```python
from build123d import *

# Parameters (mm, degrees)
BOSS_EXTRUDE1_DEPTH = 609.6
SKETCH3_W           = 635.2
SKETCH3_H           = 38.1
CUT_EXTRUDE1_DEPTH  = 60


with BuildPart() as part:
    # Sketch2 → Boss-Extrude1 (new, symmetric)
    with BuildSketch(Plane.XY):
        with BuildLine():
            Line((-19.05, -19.05), (19.05, -19.05))
            Line((19.05, -19.05), (19.05, 19.05))
            Line((19.05, 19.05), (17.4625, 19.05))
            ThreePointArc((17.4625, 19.05), (16.339967985, 18.585032015), (15.875, 17.4625))
            Line((15.875, 17.4625), (15.875, -11.0998))
            ThreePointArc((15.875, -11.0998), (14.476376302, -14.476376302), (11.0998, -15.875))
            Line((11.0998, -15.875), (-17.4625, -15.875))
            ThreePointArc((-17.4625, -15.875), (-18.585032015, -16.339967985), (-19.05, -17.4625))
            Line((-19.05, -17.4625), (-19.05, -19.05))
        make_face()
    extrude(amount=BOSS_EXTRUDE1_DEPTH, both=True)

    # Sketch3 → Cut-Extrude1 (cut)
    with BuildSketch(Plane(origin=(19.05, 0, 0), x_dir=(0, 0, -1), z_dir=(1, 0, 0))):
        with Locations((292, 0)):
            Rectangle(SKETCH3_W, SKETCH3_H)
    extrude(amount=-CUT_EXTRUDE1_DEPTH, mode=Mode.SUBTRACT)


solid = part.part
```
Work out the finished part from the listing and answer in its coordinate system (mm). A direction names the side the tool comes from. Coordinates: 2 decimals unless noted, no trailing zeros. Write each loop counter-clockwise with the first axis right and the second up, starting at its lowest first coordinate (ties: lowest second). Pieces come first, ordered by that corner, then holes.
Q1. Find the intervals of material crossed by line 1 (Y direction, x = -17, z = 427) (3 decimals); line 2 (X direction, y = 3, z = 60) (3 decimals); line 3 (X direction, y = -12, z = 65), in increasing order.
Q2. A cutting plane is placed at C-C, the plane x = -0.5. Give the vertices of the cut face in (y, z) (3 decimals).
Q3. A cutting plane is placed at B-B, the plane y = 3. Give the vertices of the cut face in (x, z) (3 decimals).
Q4. Each of these flat-tipped pins is pushed along its axis until it touches: pin 1 Ø6 at (x, z) = (-13.5, 237) entering from +Y (3 decimals); pin 2 Ø3 at (y, z) = (6, 534) entering from -X (3 decimals). Where does it stop, or does it pass through?
Q5. Which of the six approach directions +Z, -Z, +X, -X, +Y, -Y give full straight-line access (tool end or side, diameter ignored) to faces 1 (the face through (19.05, 0, 322)), 2 (the face through (-3, -15.875, 322))?
Findings below:
1. line 1: y = -19.05 to -15.875
1. line 2: x = 15.875 to 19.05
1. line 3: x = 15.79 to 19.05
2. outline: (-19.05, 25.6) - (-15.875, 25.6) - (-15.875, 609.6) - (-19.05, 609.6) - close
3. outline: (15.875, 25.6) - (19.05, 25.6) - (19.05, 609.6) - (15.875, 609.6) - close
4. pin 1: stops at y = -15.875
4. pin 2: stops at x = 15.875
5. face 1: +Z, -Z, +X, +Y, -Y
5. face 2: +Z, -Z, -X, +Y
